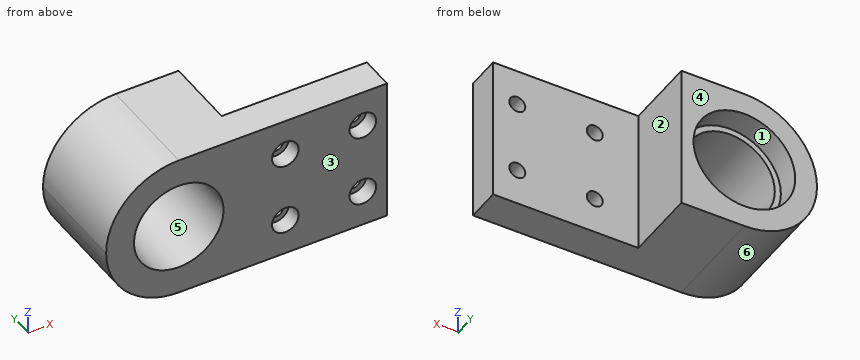
from build123d import *

# Parameters (mm, degrees)
EXTRUDE_1_DEPTH              = 60
FILLET_1_R                   = 30
SKETCH_2_R                   = 21
CUT_EXTRUDE_1_DEPTH          = 10
CUT_EXTRUDE_2_DEPTH          = 135.951843263
CUT_EXTRUDE_2_DEPTH_BACK     = 135.951843263
SKETCH_3_R                   = 18.5
HOLE_WIZARD_M6_1_D           = 6.6
HOLE_WIZARD_M6_1_CBORE_D     = 11
HOLE_WIZARD_M6_1_CBORE_DEPTH = 6.8


with BuildPart() as part:
    # 草图1 → 凸台-拉伸1 (new body)
    with BuildSketch(Plane.XY):
        Polygon((0, 0), (-116, 0), (-116, 44), (-60, 44), (-60, 14), (0, 14), align=None)
    extrude(amount=EXTRUDE_1_DEPTH)

    # 圆角1
    fillet_1_edges = [part.edges().sort_by_distance(p)[0] for p in [
        (-116, 22, 60),
        (-116, 22, 0),
    ]]
    fillet(fillet_1_edges, radius=FILLET_1_R - 0.0001)  # a hair under: the kernel refuses the full size

    # 草图2 → 切除-拉伸1 (cut)
    with BuildSketch(Plane(origin=(0, 44, 0), x_dir=(1, 0, 0), z_dir=(0, 1, 0))):
        with Locations(Location((-86, -30, 0), (0, 0, 180))):
            Circle(SKETCH_2_R)
    extrude(amount=-CUT_EXTRUDE_1_DEPTH, mode=Mode.SUBTRACT)

    # 草图3 → 切除-拉伸2 (cut, two sides: drawn at the far end of the back side and taken through both)
    with BuildSketch(Plane(origin=(0, 34, 0), x_dir=(1, 0, 0), z_dir=(0, 1, 0)).offset(-CUT_EXTRUDE_2_DEPTH_BACK)):
        with Locations(Location((-86, -30, 0), (0, 0, 180))):
            Circle(SKETCH_3_R)
    extrude(amount=CUT_EXTRUDE_2_DEPTH + CUT_EXTRUDE_2_DEPTH_BACK, mode=Mode.SUBTRACT)

    # M6 六角圆柱头螺钉的柱形沉头孔1 (through all)
    with Locations(Plane.XZ):
        with Locations((-10, 45), (-42, 15), (-42, 45), (-10, 15)):
            CounterBoreHole(HOLE_WIZARD_M6_1_D / 2, HOLE_WIZARD_M6_1_CBORE_D / 2, HOLE_WIZARD_M6_1_CBORE_DEPTH)


solid = part.part
Could you check a few things on this model? Use its own coordinates, in mm. Face numbers are marked on the shaded views. A direction names the side the tool comes from. Give positions to 0.01 mm unless a question says otherwise; leave off trailing zeros. Order: outer loops, then holes, each group sorted by start corner. A loop starts at its lowest first (then second) coordinate and runs counter-clockwise, first axis right, second up. Notation, with made-up numbers: (5, 82.25) -> (25, 82.25) arc R21 cw to (25, 113.25) -> close; hole circle Ø7 at (3, 40). An arc over 180 degrees is marked (long way). Return JSON: item names as keys, results as strings.
1. Thinking about a two-plate mould opening in Z: for the marked faces 4, 5 and 6, which applies, pulls with the +Z half, pulls with the -Z half, needs draft (parallel to the pull), parting line crosses it, or undercut?
Answer list:
{"face 4": "needs draft", "face 5": "undercut", "face 6": "pulls with the -Z half"}
2. Imagine slicing it at C-C on z = 13.5. Give the number of separate pieces and of enclosed holes in the cut face, then the cut area to 3 significant figures.
Answer list:
{"separate pieces": "4", "enclosed holes": "0", "area": "2,030 mm2"}
3. I need wall thicknesses on line 1 (Z direction, x = -42, y = 8); line 2 (Z direction, x = -42, y = 4.25); line 3 (Z direction, x = -81.5, y = 42). Which ranges of each line are inside material? Lowest first, please. Write a range as from..to.
Answer list:
{"line 1": "z = 0..11.7, 18.3..41.7, 48.3..60", "line 2": "z = 0..9.5, 20.5..39.5, 50.5..60", "line 3": "z = 0..9.49, 50.51..60"}
4. On a 3-axis mill with a long thin cutter (end or side, diameter ignored), from which of +Z, -Z, +X, -X, +Y, -Y can I reach the whole of each face in a straight line? I mean the marked faces 1, 2 and 3. Say none if no direction works.
Answer list:
{"face 1": "+Y", "face 2": "+Z, -Z, +X, +Y", "face 3": "+Z, -Z, +X, -X, -Y"}
5. For pin 1 Ø5 at (x, z) = (-42.5, 21.5) entering from +Y; pin 2 Ø10 at (y, z) = (28, 50) entering from +X; pin 3 Ø10 at (x, z) = (-42, 15) entering from -Y, each with a flat end and sliding along its axis, tell me the tip position at first contact or that it passes through.
Answer list:
{"pin 1": "stops at y = 14", "pin 2": "stops at x = -60", "pin 3": "stops at y = 6.8"}
6. Imagine slicing it at B-B on x = -10. List the corners of the cut face in (y, z) for me.
Answer list:
{"outline": "(0, 0) -> (14, 0) -> (14, 11.7) -> (6.8, 11.7) -> (6.8, 9.5) -> (0, 9.5) -> close; (0, 20.5) -> (6.8, 20.5) -> (6.8, 18.3) -> (14, 18.3) -> (14, 41.7) -> (6.8, 41.7) -> (6.8, 39.5) -> (0, 39.5) -> close; (0, 50.5) -> (6.8, 50.5) -> (6.8, 48.3) -> (14, 48.3) -> (14, 60) -> (0, 60) -> close"}
